Verification items for the finished model (mm, model axes). A direction names the side the tool comes from. Give positions to 0.01 mm unless a question says otherwise; leave off trailing zeros. Order: outer loops, then holes, each group sorted by start corner. A loop starts at its lowest first (then second) coordinate and runs counter-clockwise, first axis right, second up. Notation, with made-up numbers: (73, 36.5) - (120, 36.5) arc R10 cw to (120, 42.5) - close; hole circle Ø10 at (58, 57.5). An arc over 180 degrees is marked (long way). Answer as a JSON object with one key per item and string values. Group by question number.
(1) Section check C-C (z = -7). Record the boundary of the cut face in (x, y).
(2) Access from +Z, -Z, +X, -X, +Y, -Y to the whole of each face (thin tool, end or side, straight path). Record for faces 1 (the face through (13, 14, -28.72)), 2 (the face through (12, 20, -34)).
(3) Depth check by flat-ended pin: pin 1 Ø7.5 at (x, z) = (10, -20.5) entering from +Y; pin 2 Ø4 at (x, y) = (14, 14) entering from +Z; pin 3 Ø10 at (y, z) = (17, -9.5) entering from +X. Enter the tip coordinate at first touch or a pass-through.
(4) Section check A-A (x = 4.5). Record the boundary of the cut face in (y, z).
(5) Thickness scan on line 1 (Y direction, x = 15.75, z = -4.5); line 2 (Z direction, x = 18.5, y = 16.75). Record the ranges inside material, lowest first.
(6) Section check B-B (y = 11.75). Record the boundary of the cut face in (x, z), then the cut area to 3 significant figures.
Autodesk Inventor part; units mm, degrees
ref_plane "YZ Plane" through (0, 0, 0) normal (1, 0, 0) x (0, 1, 0)
ref_plane "XZ Plane" through (0, 0, 0) normal (0, 1, 0) x (-1, 0, 0)
ref_plane "XY Plane" through (0, 0, 0) normal (0, 0, 1) x (1, 0, 0)
sketch "Esboço1" plane through (0, 0, 0) normal (1, 0, 0) x (0, 1, 0)
  line L0 (0, 0) -> (20, 0)
  line L1 (20, 0) -> (20, -40)
  line L2 (20, -40) -> (0, -40)
  line L3 (0, -40) -> (0, 0)
  dimension "d0" = 40
  dimension "d1" = 20
extrude "Extrusão1" add sketch "Esboço1" along normal blind 25
sketch "Esboço2" plane through (25, 0, 0) normal (1, 0, 0) x (0, 0, -1)
  line L0 (28.7205, 20) -> (-11.2795, 20)
  line L1 (-11.2795, 20) -> (-11.2795, 7.5964)
  line L2 (-11.2795, 7.5964) -> (28.7205, 7.5964)
  line L3 (28.7205, 7.5964) -> (28.7205, 20)
  line L4 (0, 0) -> (40, 0)
  dimension "d4" = 40
  dimension "d5" = 20
extrude "Extrusão2" cut sketch "Esboço2" against normal through all
properties part number "Peça_aula"
Solutions:
{
 "1": {"outline": "(0, 0) - (25, 0) - (25, 7.6) - (0, 7.6) - close"},
 "2": {"face 1": "+Z, +X, -X, +Y", "face 2": "+Z, -Z, +X, -X, +Y"},
 "3": {"pin 1": "stops at y = 7.6", "pin 2": "stops at z = -28.72", "pin 3": "passes through"},
 "4": {"outline": "(0, -40) - (20, -40) - (20, -28.72) - (7.6, -28.72) - (7.6, 0) - (0, 0) - close"},
 "5": {"line 1": "y = 0 to 7.6", "line 2": "z = -40 to -28.72"},
 "6": {"outline": "(0, -40) - (25, -40) - (25, -28.72) - (0, -28.72) - close", "area": "282 mm2"}
}
